from build123d import *

# Parameters (mm, degrees)
BOSS_EXTRU_1_DEPTH = 2


with BuildPart() as part:
    # Esquisse1 → Boss.-Extru.1 (new body)
    with BuildSketch(Plane(origin=(0, 0, 0), x_dir=(1, 0, 0), z_dir=(0, 1, 0))):
        with BuildLine():
            Line((-72.21150364, 21.327505301), (85.019264112, 21.327505301))
            Line((85.019264112, 21.327505301), (85.019264112, -18.672494699))
            ThreePointArc((85.019264112, -18.672494699), (46.232543926, 9.298568327), (6.403880236, -17.167779708))
            ThreePointArc((6.403880236, -17.167779708), (-33.424783453, 9.298568327), (-72.21150364, -18.672494699))
            Line((-72.21150364, -18.672494699), (-72.21150364, 21.327505301))
        make_face()
    extrude(amount=BOSS_EXTRU_1_DEPTH)


solid = part.part
Build history of the part. All positions in model axes, mm. Round coordinates to 2 decimals unless told otherwise and drop trailing zeros. Loops run counter-clockwise (first coordinate to the right, second up) from the corner with the lowest first, then second, coordinate; pieces in that order, holes last. Notation, with made-up numbers: (45.5, -3) -> (52.5, -3) arc R25 ccw to (52.5, 30) -> close; hole circle Ø2 at (89.25, 69.25). An arc over 180 degrees is marked (long way). Use CSV: the item, a comma, the result in double quotes. Start each with the question number.
Q1. Saw through at D-D on x = -28. Give the cut face in (y, z), and give its area (3 significant figures).
Q2. Saw through at A-A on z = -8. Give the cut face in (x, y), and give its area (3 significant figures).
Q3. Flat gauge pins, fed straight in: pin 1 Ø3 at (x, z) = (64.5, -1.5) entering from -Y; pin 2 Ø1 at (x, y) = (49, 1) entering from +Z. Where does each tip first touch, or does it go through?
Q4. Drill centre lines: L1, parallel to X at y = 0.2, z = 2; L2, parallel to X at y = 1.7, z = 3; L3, parallel to Z at x = -32, y = 1.8. Where is each one in solid material? Low to high.
Q5. Saw through at B-B on y = 1.6. Give the cut face in (x, z), and give its area (3 significant figures).
Q6. Saw through at C-C on z = 8. Give the cut face in (x, y) (1 decimal), and give its area (3 significant figures).
Q7. Mould opens along X. For faces 1 (the face through (-32.713, 0.986, -9.306)), 2 (the face through (8, 2, -10)) say: +X half, -X half, draft (parallel to the pull), parting line (faces both ways), or undercut.
Solutions:
1,outline,"(0, -21.33) -> (2, -21.33) -> (2, -9.05) -> (0, -9.05) -> close"
1,area,"24.6 mm^2"
2,outline,"(-72.21, 0) -> (-43.01, 0) -> (-43.01, 2) -> (-72.21, 2) -> close; (-22.23, 0) -> (35.04, 0) -> (35.04, 2) -> (-22.23, 2) -> close; (55.82, 0) -> (85.02, 0) -> (85.02, 2) -> (55.82, 2) -> close"
2,area,"231 mm^2"
3,pin 1,"passes through"
3,pin 2,"stops at z = -9.11"
4,L1,"x = -72.21 to -61.29, -3.95 to 16.76, 74.1 to 85.02"
4,L2,"x = -72.21 to -62.32, -2.92 to 15.73, 75.13 to 85.02"
4,L3,"z = -21.33 to -9.3"
5,outline,"(-72.21, -21.33) -> (85.02, -21.33) -> (85.02, 18.67) arc R42 cw to (6.4, 17.17) arc R42 cw to (-72.21, 18.67) -> close"
5,area,"3,060 mm^2"
6,outline,"(-72.2, 0) -> (-66.6, 0) -> (-66.6, 2) -> (-72.2, 2) -> close; (1.4, 0) -> (11.5, 0) -> (11.5, 2) -> (1.4, 2) -> close; (79.4, 0) -> (85, 0) -> (85, 2) -> (79.4, 2) -> close"
6,area,"42.7 mm^2"
7,face 1,"undercut"
7,face 2,"draft"
